Autodesk Inventor part; units mm, degrees
ref_plane "YZ Plane" through (0, 0, 0) normal (1, 0, 0) x (0, 1, 0)
ref_plane "XZ Plane" through (0, 0, 0) normal (0, 1, 0) x (-1, 0, 0)
ref_plane "XY Plane" through (0, 0, 0) normal (0, 0, 1) x (1, 0, 0)
sketch "Sketch1" plane through (0, 0, 0) normal (0, 0, 1) x (1, 0, 0)
  line L0 (0, 0) -> (35.08, 0)
  line L1 (35.08, 0) -> (35.08, -60)
  line L2 (35.08, -60) -> (0, -60)
  line L3 (0, -60) -> (0, 0)
  dimension "d0" = 35.08
  dimension "d1" = 60
extrude "Extrusion1" add sketch "Sketch1" along normal blind 4
sketch "Sketch2" plane through (0, 0, 4) normal (0, 0, 1) x (1, 0, 0)
  line L0 (35.08, 0) -> (0, 0)
  line L1 (2, -2) -> (33.08, -2)
  line L2 (33.08, -2) -> (33.08, -58)
  line L3 (33.08, -58) -> (2, -58)
  line L4 (2, -58) -> (2, -2)
  line L5 (0, -60) -> (35.08, -60)
  line L6 (35.08, -60) -> (35.08, 0)
  line L7 (0, 0) -> (0, -60)
  dimension "d8" = 2
  dimension "d9" = 2
  dimension "d10" = 2
  dimension "d11" = 2
extrude "Extrusion2" cut sketch "Sketch2" against normal blind 2 contours L1 L2 L3 L4
properties part number "tapaBateria"
The model under review builds one solid part; all positions refer to its coordinate system, in mm. A direction names the side the tool comes from. Round coordinates to 2 decimals unless told otherwise and drop trailing zeros. Loops run counter-clockwise (first coordinate to the right, second up) from the corner with the lowest first, then second, coordinate; pieces in that order, holes last. Notation, with made-up numbers: M 58.5,40 L 78.5,40 A20 cw 78.5,63 Z; hole C 42.5,-29.5 d9. An arc over 180 degrees is marked long. Answer as CSV lines item,"result". Start each with the question number.
Item 1: Insertion check: P1, Ø2, axis at x = 22.5, y = -17, coming from the +Z side. The pin has a flat end and moves straight along its axis. Give the tip position at first contact, or say it passes through.
Item 2: Consider section C-C (y = -40.5). Write out the cut boundary in (x, z).
Item 3: Consider section A-A (x = 10). Write out the cut boundary in (y, z), then the cut area to 3 significant figures.
Item 4: Mouldability with a two-part tool opening along Y and no side actions: class faces 3 (the face through (0, -30, 2)), 4 (the face through (17, 0, 2)), 5 (the face through (2, -30, 3)) as released by +Y, released by -Y, zero draft, split by the parting line, or undercut.
Item 5: For faces 1 (the face through (33.08, -30, 3)), 2 (the face through (17, -30, 0)), list the 3-axis set-ups (+Z, -Z, +X, -X, +Y, -Y) from which the entire face can be reached by the end or side of a thin tool; tool diameter is ignored.
Item 6: Consider section B-B (z = 3.15). Write out the cut boundary in (x, y), then the cut area to 3 significant figures.
Item 7: Wall thickness on line 1 (X direction, y = -4, z = 3.55); line 2 (Y direction, x = 33, z = 3.6); line 3 (Z direction, x = 23, y = -50): over which ranges is each line inside the solid? List them lowest first. Write a range as [from, to].
Answer:
1,P1,"stops at z = 2"
2,outline,"M 0,0 L 35.08,0 L 35.08,4 L 33.08,4 L 33.08,2 L 2,2 L 2,4 L 0,4 Z"
3,outline,"M -60,0 L 0,0 L 0,4 L -2,4 L -2,2 L -58,2 L -58,4 L -60,4 Z"
3,area,"128 mm^2"
4,face 3,"zero draft"
4,face 4,"released by +Y"
4,face 5,"undercut"
5,face 1,"+Z"
5,face 2,"-Z, +X, -X, +Y, -Y"
6,outline,"M 0,-60 L 35.08,-60 L 35.08,0 L 0,0 Z; hole M 2,-58 L 33.08,-58 L 33.08,-2 L 2,-2 Z"
6,area,"364 mm^2"
7,line 1,"x = [0, 2], [33.08, 35.08]"
7,line 2,"y = [-60, -58], [-2, 0]"
7,line 3,"z = [0, 2]"
